Could you check a few things on this model? Use its own coordinates, in mm. Face numbers are marked on the shaded views. Give positions to 0.01 mm unless a question says otherwise; leave off trailing zeros. Order: outer loops, then holes, each group sorted by start corner. A loop starts at its lowest first (then second) coordinate and runs counter-clockwise, first axis right, second up. Notation, with made-up numbers: M 26,2.25 L 66,2.25 A17 cw 66,22.25 Z; hole C 37,7 d9. An arc over 180 degrees is marked long. Answer in a Markdown table with one row per item. Add a question column.
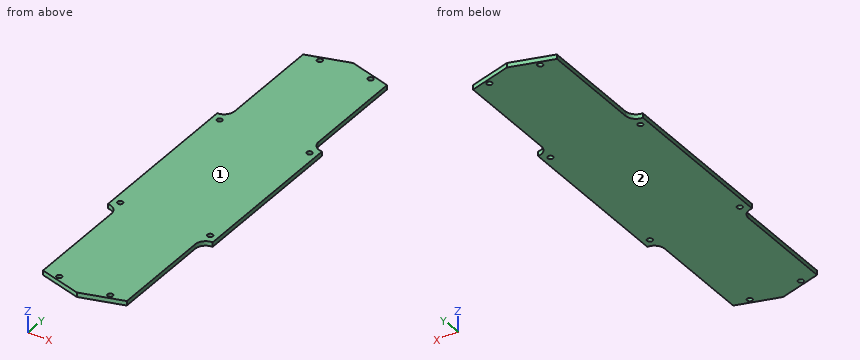
Autodesk Fusion 360 part; units mm, degrees
sketch "Skizze1" plane through (0, 0, 0) normal (0, 0, 1) x (1, 0, 0)
  line L0 (-48.5045, 60.0252) -> (-48.5045, -50)
  line L1 (21.4307, 60.0126) -> (21.4307, -50)
  line L2 (-41.5077, 135.8568) -> (-13.5563, 144.0233)
  line L3 (-13.5563, 144.0233) -> (14.4793, 135.8568)
  line L4 (-41.4821, -125.8001) -> (-13.5254, -133.9377)
  line L5 (-13.5254, -133.9377) -> (14.4312, -125.8001)
  line L6 (14.4312, -125.8001) -> (14.4312, -57)
  line L7 (-41.4821, -125.8001) -> (-41.4821, -57)
  line L8 (-41.5077, 135.8568) -> (-41.5077, 66.6867)
  line L9 (14.4793, 135.8568) -> (14.4793, 66.6867)
  circle A0 centre (3.4202, 136.0177) radius 1.7651
  circle A1 centre (-30.4724, 136.0177) radius 1.7717
  circle A2 centre (-30.5621, -125.8912) radius 1.7405
  circle A3 centre (3.437, -125.8912) radius 1.7197
  circle A4 centre (-43.5796, -44.9629) radius 1.7343
  circle A5 centre (16.4191, -44.9629) radius 1.761
  circle A6 centre (-43.5796, 55.0289) radius 1.7075
  circle A7 centre (16.4191, 55.0289) radius 1.7507
  line L10 (21.4307, 60.0126) -> (21.4793, 60.0126)
  line L11 (14.4793, 67.0126) -> (14.4793, 66.6867)
  line L12 (-41.5077, 66.6867) -> (-41.5077, 67.0252)
  line L13 (-48.5077, 60.0252) -> (-48.5045, 60.0252)
  line L14 (-48.5045, -50) -> (-48.4821, -50)
  line L15 (21.4312, -50) -> (21.4307, -50)
  arc A8 (21.4312, -50) -> (14.4312, -57) centre (21.4312, -57) ccw
  arc A9 (-41.4821, -57) -> (-48.4821, -50) centre (-48.4821, -57) ccw
  arc A10 (-48.5077, 60.0252) -> (-41.5077, 67.0252) centre (-48.5077, 67.0252) ccw
  arc A11 (14.4793, 67.0126) -> (21.4793, 60.0126) centre (21.4793, 67.0126) ccw
  dimension "d1" = 7
  dimension "d2" = 7
  dimension "d3" = 7
  dimension "d4" = 7
extrude "Extrusion1" add sketch "Skizze1" along normal blind 3
1. If I drill on line 1 along X through (y, z) = (55, 1.4); line 2 along Y through (x, z) = (-32, 1.85); line 3 along Y through (x, z) = (3.5, 0.5), over which ranges is the centre line in solid material (lowest first)? Write a range as [from, to].
2. Suppose I cut it at C-C on x = -23.5. List the corners of the cut face in (y, z) for me, plus the area to 3 significant figures.
3. Suppose I cut it at B-B on y = 88.5. List the corners of the cut face in (x, z) for me, plus the area to 3 significant figures.
4. Thinking about a two-plate mould opening in Z: for the marked faces 1 and 2, which applies, pulls with the +Z half, pulls with the -Z half, needs draft (parallel to the pull), parting line crosses it, or undercut?
5. Suppose I cut it at A-A on z = 0.5. Count the separate pieces of the cut face and the enclosed holes in it, plus the area to 3 significant figures.
6. Will this pin go through, and if not, where does the flat tip stop? P1, Ø1, axis at y = 86.5, z = 1.5, coming from the +X side.
Findings below:
| question | item | result |
|---|---|---|
| 1 | line 1 | [-48.5, -45.29], [-41.87, 14.67], [18.17, 21.43] |
| 1 | line 2 | [-128.56, -126.87], [-124.91, 135.12], [136.92, 138.63] |
| 1 | line 3 | [-128.98, -127.61], [-124.17, 134.25], [137.78, 139.05] |
| 2 | outline | M -131.03,0 L 141.12,0 L 141.12,3 L -131.03,3 Z |
| 2 | area | 816 mm2 |
| 3 | outline | M -41.51,0 L 14.48,0 L 14.48,3 L -41.51,3 Z |
| 3 | area | 168 mm2 |
| 4 | face 1 | pulls with the +Z half |
| 4 | face 2 | pulls with the -Z half |
| 5 | separate pieces | 1 |
| 5 | enclosed holes | 8 |
| 5 | area | 16,600 mm2 |
| 6 | P1 | x = 14.48 |
